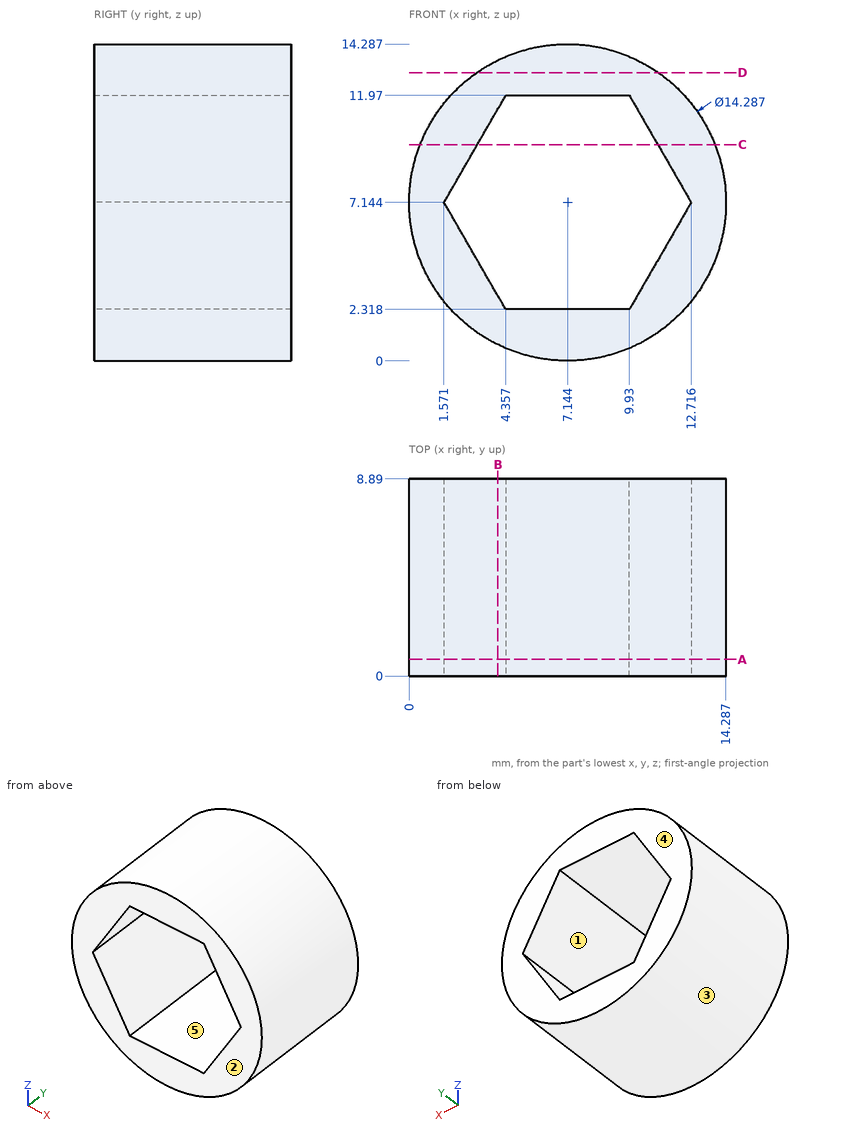
Geometry check sheet. Reference: drawing and pictorial views, mm from the part's lowest x, y, z. A direction names the side the tool comes from. Give positions to 0.01 mm unless a question says otherwise; leave off trailing zeros. Write each loop counter-clockwise with the first axis right and the second up, starting at its lowest first coordinate (ties: lowest second). Pieces come first, ordered by that corner, then holes. Notation, with made-up numbers: (32.25, 12.25) -> (36.25, 12.25) arc R25 ccw to (36.25, 48.25) -> close; hole circle Ø3 at (-20.75, -39.5). An arc over 180 degrees is marked (long way). One line per item, written item: value. Start each with the question number.
Item 1: Draft check along Z on the marked faces 3, 4 and 5. Enter one of: +Z half, -Z half, draft (parallel to the pull), parting line (faces both ways), or undercut.
Item 2: Gauge pin test, flat ends, axial feed: pin 1 (1.5 mm diameter, centred on x = 8, y = 2.5, fed in from +Z); pin 2 (2 mm diameter, centred on x = 4, y = 2, fed in from -Z); pin 3 (2 mm diameter, centred on x = 4.5, z = 5, fed in from +Y). Record the tip position at first contact, or that the pin passes through.
Item 3: Section check A-A on y = 0.75. Record the cut outline in (x, z).
Item 4: Section check D-D on z = 13. Record the cut outline in (x, y) (1 decimal).
Item 5: Material ranges on probe 1 along Z at (x, y) = (7, 3.75); probe 2 along Z at (x, y) = (8, 6.5) (1 decimal); probe 3 along X at (y, z) = (3.75, 6.5) (1 decimal), recorded low to high. Write a range as from..to.
Item 6: Section check C-C on z = 9.75. Record the cut outline in (x, y) (1 decimal).
Item 7: Section check B-B on x = 4. Record the cut outline in (y, z).
Item 8: Tool access check on the marked faces 1 and 2. Record the directions out of +Z, -Z, +X, -X, +Y, -Y that give a thin tool (end or side, any length) a straight path to the whole face; none if there is none.
Results list:
1. face 3: parting line
1. face 4: draft
1. face 5: undercut
2. pin 1: z = 14.29
2. pin 2: z = 0.33
2. pin 3: through
3. outline: circle Ø14.29 at (7.14, 7.14); hole (1.57, 7.14) -> (4.36, 2.32) -> (9.93, 2.32) -> (12.72, 7.14) -> (9.93, 11.97) -> (4.36, 11.97) -> close
4. outline: (3.1, 0) -> (11.2, 0) -> (11.2, 8.9) -> (3.1, 8.9) -> close
5. probe 1: 0..2.32, 11.97..14.29
5. probe 2: 0.1..2.3, 12..14.2
5. probe 3: 0..1.9, 12.3..14.3
6. outline: (0.5, 0) -> (3.1, 0) -> (3.1, 8.9) -> (0.5, 8.9) -> close; (11.2, 0) -> (13.8, 0) -> (13.8, 8.9) -> (11.2, 8.9) -> close
7. outline: (0, 0.73) -> (8.89, 0.73) -> (8.89, 2.94) -> (0, 2.94) -> close; (0, 11.35) -> (8.89, 11.35) -> (8.89, 13.56) -> (0, 13.56) -> close
8. face 1: +Y, -Y
8. face 2: +Z, -Z, +X, -X, -Y
